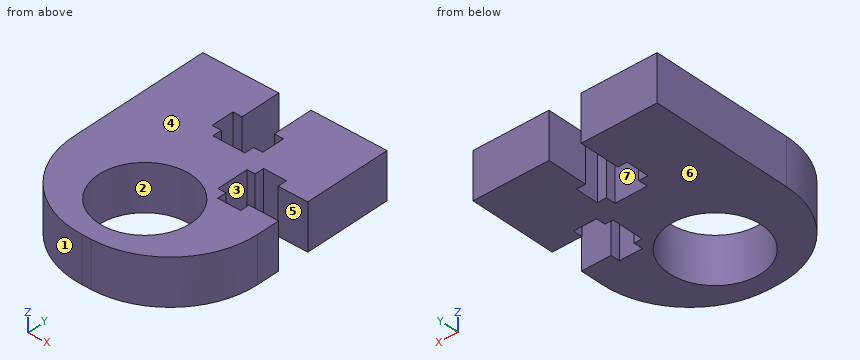
Autodesk Inventor part; units mm, degrees
ref_plane "YZ Plane" through (0, 0, 0) normal (1, 0, 0) x (0, 1, 0)
ref_plane "XZ Plane" through (0, 0, 0) normal (0, 1, 0) x (-1, 0, 0)
ref_plane "XY Plane" through (0, 0, 0) normal (0, 0, 1) x (1, 0, 0)
sketch "Boceto1" plane through (0, 0, 0) normal (0, 0, 1) x (1, 0, 0)
  line L0 (0, 0) -> (20, 0)
  line L1 (20, 0) -> (20, -25)
  line L2 (20, -25) -> (0, -25)
  line L3 (0, -25) -> (0, 0)
  circle A0 centre (10, -18) radius 5
  dimension "d0" = 20
  dimension "d1" = 25
  dimension "d2" = 7
extrude "Extrusión1" add sketch "Boceto1" along normal blind 5
sketch "Boceto2" plane through (0, 0, 5) normal (0, 0, 1) x (1, 0, 0)
  line L0 (0, 0) -> (20, 0)
  line L1 (11.75, -7.9211) -> (8.25, -7.9211)
  line L2 (7.25, -4.3971) -> (7.25, -6.8971)
  line L3 (12.75, -6.8971) -> (12.75, -4.3971)
  line L4 (7.25, -6.8971) -> (8.25, -6.8971)
  line L5 (11.75, -6.8971) -> (12.75, -6.8971)
  line L6 (12.75, -4.3971) -> (11.75, -4.3971)
  line L7 (8.25, -4.3971) -> (7.25, -4.3971)
  line L8 (8.25, -7.9211) -> (8.25, -6.8971)
  line L9 (8.25, -4.3971) -> (8.25, 0)
  line L10 (11.75, 0) -> (11.75, -4.3971)
  line L11 (11.75, -6.8971) -> (11.75, -7.9211)
extrude "Extrusión2" cut sketch "Boceto2" against normal through all
sketch "Boceto3" plane through (0, 0, 5) normal (0, 0, 1) x (1, 0, 0)
  line L0 (20, 0) -> (20, -25)
  line L1 (13.4106, -9.5) -> (13.4106, -13)
  line L2 (14.2856, -8.5) -> (16.7856, -8.5)
  line L3 (16.7856, -14) -> (14.2856, -14)
  line L4 (16.7856, -8.5) -> (16.7856, -9.5)
  line L5 (16.7856, -13) -> (16.7856, -14)
  line L6 (14.2856, -14) -> (14.2856, -13)
  line L7 (14.2856, -9.5) -> (14.2856, -8.5)
  line L8 (20, -9.5) -> (16.7856, -9.5)
  line L9 (14.2856, -9.5) -> (13.4106, -9.5)
  line L10 (13.4106, -13) -> (14.2856, -13)
  line L11 (16.7856, -13) -> (20, -13)
  dimension "d12" = 5.5
extrude "Extrusión3" cut sketch "Boceto3" against normal through all
fillet "Empalme1" radius 9.5 2 edges at (0, -25, 2.5) (20, -25, 2.5)
properties part number "soporte polea eje x"
Could you check a few things on this model? Use its own coordinates, in mm. Face numbers are marked on the shaded views. A direction names the side the tool comes from. Give positions to 0.01 mm unless a question says otherwise; leave off trailing zeros. Order: outer loops, then holes, each group sorted by start corner. A loop starts at its lowest first (then second) coordinate and runs counter-clockwise, first axis right, second up. Notation, with made-up numbers: (-4.5, 84) - (11.5, 84) arc R28 cw to (11.5, 104) - close; hole circle Ø10 at (-35.75, 25.25). An arc over 180 degrees is marked (long way). Return JSON: item names as keys, results as strings. Group by question number.
Q1. Thinking about a two-plate mould opening in Y: for the marked faces 1, 2, 3 and 4, which applies, pulls with the +Y half, pulls with the -Y half, needs draft (parallel to the pull), parting line crosses it, or undercut?
Q2. Which directions (+Z, -Z, +X, -X, +Y, -Y) give clear straight access to the entire face, cutting with the end or side of a thin tool? Please do the marked faces 5, 6 and 7.
Q3. Will these pins go through, and if not, where does the flat tip stop? pin 1 Ø1.8 at (y, z) = (-12, 2.5) entering from +X; pin 2 Ø1.5 at (x, z) = (2, 3.5) entering from -Y; pin 3 Ø2.5 at (x, z) = (18, 2.5) entering from -Y.
Q4. Suppose I cut it at C-C, the plane y = -3.5. Please give me the cut outline in (x, z).
Q5. Suppose I cut it at B-B, the plane x = 10. Please give me the cut outline in (y, z), and give its area (3 significant figures).
Q6. Suppose I cut it at D-D, the plane x = 3.25. Please give me the cut outline in (y, z).
Q7. Please list where these lines run through material, in increasing order: line 1 along X through (y, z) = (-7.5, 1.85); line 2 along Y through (x, z) = (7.75, 2.8); line 3 along X through (y, z) = (-5.5, 3.95). Write a range as [from, to].
Resolved:
{
 "1": {"face 1": "pulls with the -Y half", "face 2": "undercut", "face 3": "undercut", "face 4": "needs draft"},
 "2": {"face 5": "+Z, -Z, +X", "face 6": "-Z, +X, -X, +Y, -Y", "face 7": "+Z, -Z, +Y"},
 "3": {"pin 1": "stops at x = 13.41", "pin 2": "stops at y = -22.18", "pin 3": "stops at y = -22.65"},
 "4": {"outline": "(0, 0) - (8.25, 0) - (8.25, 5) - (0, 5) - close; (11.75, 0) - (20, 0) - (20, 5) - (11.75, 5) - close"},
 "5": {"outline": "(-25, 0) - (-23, 0) - (-23, 5) - (-25, 5) - close; (-13, 0) - (-7.92, 0) - (-7.92, 5) - (-13, 5) - close", "area": "35.4 mm2"},
 "6": {"outline": "(-22.65, 0) - (0, 0) - (0, 5) - (-22.65, 5) - close"},
 "7": {"line 1": "x = [0, 8.25], [11.75, 20]", "line 2": "y = [-24.84, -22.47], [-13.53, -6.9], [-4.4, 0]", "line 3": "x = [0, 7.25], [12.75, 20]"}
}
